```python
from build123d import *

# Parameters (mm, degrees)
CHAMFER1_SIZE = 1
THREAD1_PITCH = 1


with BuildPart() as part:
    # Sketch2 → Revolve1 (revolve)
    with BuildSketch(Plane(origin=(0, 0, 0), x_dir=(1, 0, 0), z_dir=(0, 1, 0)), mode=Mode.PRIVATE) as revolve1_sk:
        Polygon((0, 0), (3.75, 0), (3.75, 6.8), (4.3, 6.8), (4.7, 7.2), (4.7, 9), (3.5, 9), (3.5, 15), (2.25, 15), (2.25, 6), (0, 6), align=None)
    revolve(revolve1_sk.sketch.rotate(Axis((0, 0, -6), (0, 0, 1)), 180), axis=Axis((0, 0, -6), (0, 0, 1)))

    # Chamfer1
    chamfer1_edges = [part.edges().sort_by_distance(p)[0] for p in [
        (3.5, 0, -15),
    ]]
    chamfer(chamfer1_edges, length=CHAMFER1_SIZE)

    # Thread1: the profile of Thread Profile1 profile screwed along a right-hand helix of 4.5 turns, 8 arcs to a turn; built about Z, then put on its axis
    thread1_z = Axis((0, 0, 0), (0, 0, 1))
    thread1_corners = [(3.5003, 0, -0.000173205), (3.5003, 0, 0.875173202), (2.958734125, 0, 0.562499999), (2.958734125, 0, 0.312499999)]
    with BuildLine(mode=Mode.PRIVATE) as thread1_profile:
        Line(thread1_corners[0], thread1_corners[1])
        Line(thread1_corners[1], thread1_corners[2])
        Line(thread1_corners[2], thread1_corners[3])
        Line(thread1_corners[3], thread1_corners[0])
    thread1_cap = Face(thread1_profile.wire())
    thread1_turn_angles = [0, 22.5, 45, 67.5, 90, 112.5, 135, 157.5, 180, 202.5, 225, 247.5, 270, 292.5, 315, 337.5, 360]
    thread1_turn_weights = [1, 0.9238795325112867, 1, 0.9238795325112867, 1, 0.9238795325112867, 1, 0.9238795325112867, 1, 0.9238795325112867, 1, 0.9238795325112867, 1, 0.9238795325112867, 1, 0.9238795325112867, 1]
    thread1_turn_rails = [Edge.make_bspline([Vector(p[0], p[1], 0).rotate(thread1_z, thread1_turn_angles[k]) / thread1_turn_weights[k] + Vector(0, 0, p[2] + THREAD1_PITCH * thread1_turn_angles[k] / 360) for k in range(17)], [0, 0, 0, 1, 1, 2, 2, 3, 3, 4, 4, 5, 5, 6, 6, 7, 7, 8, 8, 8], 2, thread1_turn_weights) for p in thread1_corners]
    thread1_turn_sides = [Face.make_surface_from_curves(thread1_turn_rails[p[0]], thread1_turn_rails[p[1]]) for p in [(0, 1), (1, 2), (2, 3), (3, 0)]]
    thread1_last_angles = [1440, 1462.5, 1485, 1507.5, 1530, 1552.5, 1575, 1597.5, 1620]
    thread1_last_weights = [1, 0.9238795325112867, 1, 0.9238795325112867, 1, 0.9238795325112867, 1, 0.9238795325112966, 1]
    thread1_last_rails = [Edge.make_bspline([Vector(p[0], p[1], 0).rotate(thread1_z, thread1_last_angles[k]) / thread1_last_weights[k] + Vector(0, 0, p[2] + THREAD1_PITCH * thread1_last_angles[k] / 360) for k in range(9)], [0, 0, 0, 1, 1, 2, 2, 3, 3, 4, 4, 4], 2, thread1_last_weights) for p in thread1_corners]
    thread1_last_sides = [Face.make_surface_from_curves(thread1_last_rails[p[0]], thread1_last_rails[p[1]]) for p in [(0, 1), (1, 2), (2, 3), (3, 0)]]
    thread1 = Plane(origin=(0, 0, -15), x_dir=(1, 0, 0), z_dir=(0, 0, 1)) * Solid(Shell([*[p.moved(Location((0, 0, THREAD1_PITCH * i))) for i in range(4) for p in thread1_turn_sides], *thread1_last_sides, thread1_cap, thread1_cap.rotate(thread1_z, 1620).moved(Location((0, 0, THREAD1_PITCH * 1620 / 360)))]))
    add(thread1, mode=Mode.SUBTRACT)


solid = part.part
```
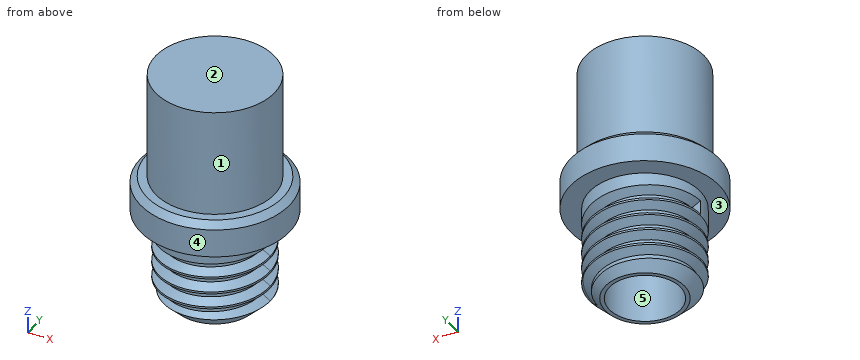
For this review, take the finished solid that the model builds, in its own axes (mm). Face numbers are marked on the shaded views. A direction names the side the tool comes from. Round coordinates to 2 decimals unless told otherwise and drop trailing zeros. Write each loop counter-clockwise with the first axis right and the second up, starting at its lowest first coordinate (ties: lowest second). Pieces come first, ordered by that corner, then holes. Notation, with made-up numbers: (61.25, -15.75) - (71.25, -15.75) arc R27 cw to (71.25, 19.25) - close; hole circle Ø7 at (59.25, -32.75). An arc over 180 degrees is marked (long way). Put each result on its own line as item: value.
Q1. We need section B-B (z = -4.75). Give the boundary of the cut face in (x, y).
Solved:
outline: circle Ø7.5 at (0, 0)
Q2. We need section A-A (z = -8). Give the boundary of the cut face in (x, y).
Solved:
outline: circle Ø9.4 at (0, 0); hole circle Ø4.5 at (0, 0)
Q3. Mouldability with a two-part tool opening along Z and no side actions: class the marked faces 1, 2 and 3 as released by +Z, released by -Z, zero draft, split by the parting line, or undercut.
Solved:
face 1: zero draft
face 2: released by +Z
face 3: released by -Z
Q4. Machinability: for the marked faces 4 and 5, which of the approach directions +Z, -Z, +X, -X, +Y, -Y give a long, thin tool a straight path to every point of the face, cutting with its end or side? Answer none if there is none.
Solved:
face 4: +Z, -Z
face 5: -Z
Q5. Insertion check: pin 1 Ø1.5 at (y, z) = (3.5, -13) entering from -X; pin 2 Ø1.5 at (x, z) = (2, -10.5) entering from -Y; pin 3 Ø4 at (x, y) = (0, 0) entering from -Z. Each pin has a flat end and moves straight along its axis. Give the tip position at first contact, or say it passes through.
Solved:
pin 1: stops at x = -2.12
pin 2: stops at y = -3.26
pin 3: stops at z = -6
Q6. Wall thickness on probe 1 along Y at (x, z) = (0, -8.5); probe 2 along Y at (x, z) = (0, -9.25); probe 3 along Z at (x, y) = (0.25, 1): over which ranges is each line inside the solid? List them lowest first.
Solved:
probe 1: y = -4.7 to -2.25, 2.25 to 4.7
probe 2: y = -3.5 to -2.25, 2.25 to 3.5
probe 3: z = -6 to 0
